from build123d import *

# Parameters (mm, degrees)
BOSS_EXTRUDE1_DEPTH     = 3
CUT_EXTRUDE1_DEPTH      = 39.19685851
CUT_EXTRUDE1_DEPTH_BACK = 39.19685851
SKETCH2_R               = 1.7
CUT_EXTRUDE2_DEPTH      = 39.19685851
CUT_EXTRUDE2_DEPTH_BACK = 39.19685851
FILLET1_R               = 2


with BuildPart() as part:
    # Sketch1 → Boss-Extrude1 (new body)
    with BuildSketch(Plane(origin=(0, 0, 0), x_dir=(1, 0, 0), z_dir=(0, 1, 0))):
        Polygon((-15, 35), (0, 35), (15, 35), (15, 0), (15, -35), (0, -35), (-15, -35), (-15, 0), align=None)
    extrude(amount=BOSS_EXTRUDE1_DEPTH)

    # Sketch2 → Cut-Extrude1 (cut, two sides: drawn at the far end of the back side and taken through both)
    with BuildSketch(Plane(origin=(0, 3, 0), x_dir=(1, 0, 0), z_dir=(0, 1, 0)).offset(-CUT_EXTRUDE1_DEPTH_BACK)):
        with Locations(Location((-9, 32.5, 0), (0, 0, 270))):
            Circle(SKETCH2_R)
        with Locations(Location((9, 32.5, 0), (0, 0, 270))):
            Circle(SKETCH2_R)
        with Locations(Location((9, -32.5, 0), (0, 0, 90))):
            Circle(SKETCH2_R)
        with Locations(Location((-9, -32.5, 0), (0, 0, 90))):
            Circle(SKETCH2_R)
    extrude(amount=CUT_EXTRUDE1_DEPTH + CUT_EXTRUDE1_DEPTH_BACK, mode=Mode.SUBTRACT)

    # Sketch3 → Cut-Extrude2 (cut, two sides: drawn at the far end of the back side and taken through both)
    with BuildSketch(Plane(origin=(0, 3, 0), x_dir=(1, 0, 0), z_dir=(0, 1, 0)).offset(-CUT_EXTRUDE2_DEPTH_BACK)):
        Polygon((-12, 27), (0, 27), (12, 27), (-12, 17), align=None)
        Polygon((-12, 14.833333333), (12, 24.833333333), (12, 14.833333333), align=None)
        Polygon((-12, 13), (0, 13), (12, 13), (-12, 3), align=None)
        Polygon((-12, 0.833333333), (12, 10.833333333), (12, 0.833333333), align=None)
        Polygon((-12, -1), (0, -1), (12, -1), (-12, -11), align=None)
        Polygon((-12, -13.166666667), (12, -3.166666667), (12, -13.166666667), align=None)
        Polygon((-12, -15), (0, -15), (12, -15), (-12, -25), align=None)
        Polygon((-12, -27.166666667), (12, -17.166666667), (12, -27.166666667), align=None)
    extrude(amount=CUT_EXTRUDE2_DEPTH + CUT_EXTRUDE2_DEPTH_BACK, mode=Mode.SUBTRACT)

    # Fillet1
    fillet1_edges = [part.edges().sort_by_distance(p)[0] for p in [
        (-15, 1.5, -35),
        (15, 1.5, -35),
        (15, 1.5, 35),
        (-15, 1.5, 35),
    ]]
    fillet(fillet1_edges, radius=FILLET1_R)


solid = part.part
Model file for the job. Use its own axes, mm. A direction names the side the tool comes from. Round coordinates to 2 decimals unless told otherwise and drop trailing zeros.
1. Band-saw the part on A-A, the plane y = 1.25. Count the separate pieces of the cut face and the enclosed holes in it, and give its area (3 significant figures).
Check values:
separate pieces: 1
enclosed holes: 12
area: 1,100 mm2
2. Mould opens along X. For faces 3 (the flat face through (0, 1, -35)), 4 (the cylindrical face through (14.43, 1.52, 34.4)), 5 (the flat face through (-12, 1, 6)) say: +X half, -X half, draft (parallel to the pull), parting line (faces both ways), or undercut.
Check values:
face 3: draft
face 4: +X half
face 5: undercut
3. Wall check: probe 1 along X at (y, z) = (0.8, 32.5); probe 2 along X at (y, z) = (0.8, -31); probe 3 along X at (y, z) = (1.85, 16.5). Give the ranges that are in metal, low to high.
Check values:
probe 1: x = -15 to -10.7, -7.3 to 7.3, 10.7 to 15
probe 2: x = -15 to -9.8, -8.2 to 8.2, 9.8 to 15
probe 3: x = -15 to -12, 8.4 to 15
4. Tool access for faces 1 (the flat face through (0, 3, 0)), 2 (the flat face through (-12, 1, -22)): list every direction of +Z, -Z, +X, -X, +Y, -Y with a clear straight run to the whole face (end or side of a thin tool).
Check values:
face 1: +Z, -Z, +X, -X, +Y
face 2: +Y, -Y
